Could you check a few things on this model? Use its own coordinates, in mm. Face numbers are marked on the shaded views. A direction names the side the tool comes from. Give positions to 0.01 mm unless a question says otherwise; leave off trailing zeros. Order: outer loops, then holes, each group sorted by start corner. A loop starts at its lowest first (then second) coordinate and runs counter-clockwise, first axis right, second up. Notation, with made-up numbers: M 61,-27 L 79,-27 A18 cw 79,1 Z; hole C 45,0 d10. An arc over 180 degrees is marked long. Use a Markdown table: item, result. Add a question column.
Item 1: Suppose I cut it at D-D on x = 10.5. Write out the boundary of the cut face in (y, z).
Item 2: I'm going to push flat-ended pins straight in: pin 1 Ø0.5 at (x, y) = (0, -3) entering from +Z; pin 2 Ø8 at (x, y) = (-1.5, -1.5) entering from -Z; pin 3 Ø2.5 at (x, y) = (0.5, 8.5) entering from +Z; pin 4 Ø1.2 at (x, y) = (0, -2.5) entering from +Z. Where does each tip first touch, or does it pass through?
Item 3: If I drill on L1, parallel to Y at x = 10.5, z = 0.7; L2, parallel to Z at x = 0.75, y = 6.25; L3, parallel to Y at x = -5.75, z = -0.2, over which ranges is the centre line in solid material (lowest first)? Write a range as from..to.
Item 4: Suppose I cut it at C-C on y = -4.5. Write out the boundary of the cut face in (x, z).
Item 5: Suppose I cut it at A-A on y = 3.25. Write out the boundary of the cut face in (x, z).
Item 6: For the marked faces 1, 2 and 3, which set-ups out of +Z, -Z, +X, -X, +Y, -Y let a thin tool reach every point of the face, with its end or its side?
Item 7: If we mould it in two halves opening along Y, with no side actions, what happens to the marked faces 4, 5 and 6? For each: released by +Y, released by -Y, zero draft, split by the parting line, or undercut.
Item 8: Suppose I cut it at B-B on x = 1.5. Write out the boundary of the cut face in (y, z) (3 decimals), plus the area to 3 significant figures.
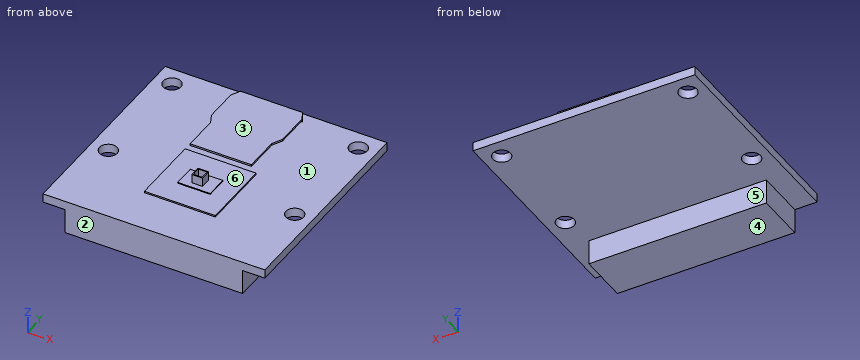
from build123d import *

# Parameters (mm, degrees)
SKETCH1_W                 = 25
SKETCH1_H                 = 24
BOSS_EXTRUDE1_DEPTH       = 1
SKETCH2_R                 = 1
CUT_EXTRUDE1_DEPTH        = 1
SKETCH3_W                 = 8
SKETCH3_H                 = 8
BOSS_EXTRUDE2_DEPTH       = 5.2
SKETCH4_W                 = 8
SKETCH4_H                 = 8
SKETCH4_R                 = 3.75
CUT_EXTRUDE2_DEPTH        = 3.2
SKETCH5_R                 = 3.75
SKETCH5_R_2               = 3
CUT_EXTRUDE3_DEPTH        = 1.2
TOP_RIBBON_DEPTH          = 1
SKETCH7_W                 = 0.8
SKETCH7_H                 = 9.7
CUT_EXTRUDE4_DEPTH        = 9
SKETCH8_W                 = 20
SKETCH8_H                 = 5.6
REAR_RIBBON_DEPTH         = 2.8
CUT_EXTRUDE5_DEPTH        = 10
CUT_EXTRUDE5_DEPTH_BACK   = 1.827942302
SKETCH9_W                 = 8
SKETCH9_H                 = 8
SKETCH10_W                = 3.67
SKETCH10_H                = 2.47
CCD_DEPTH                 = 0.1
SKETCH11_W                = 1.2
SKETCH11_H                = 1.2
SKETCH11_W_2              = 1
SKETCH11_H_2              = 1
TELESCOPE_ALIGNMENT_DEPTH = 1.1


with BuildPart() as part:
    # Sketch1 → Boss-Extrude1 (new body)
    with BuildSketch(Plane.XY):
        Rectangle(SKETCH1_W, SKETCH1_H)
    extrude(amount=BOSS_EXTRUDE1_DEPTH)

    # Sketch2 → Cut-Extrude1 (cut)
    with BuildSketch(Plane.XY.offset(1)):
        with Locations((-10.5, 9.85)):
            Circle(SKETCH2_R)
        with Locations((10.5, 9.85)):
            Circle(SKETCH2_R)
        with Locations((10.5, -2.65)):
            Circle(SKETCH2_R)
        with Locations((-10.5, -2.65)):
            Circle(SKETCH2_R)
    extrude(amount=-CUT_EXTRUDE1_DEPTH, mode=Mode.SUBTRACT)

    # Sketch3 → Boss-Extrude2 (add)
    with BuildSketch(Plane.XY.offset(1)):
        with Locations((0, -2.9)):
            Rectangle(SKETCH3_W, SKETCH3_H)
    extrude(amount=BOSS_EXTRUDE2_DEPTH)

    # Sketch4 → Cut-Extrude2 (cut)
    with BuildSketch(Plane.XY.offset(6.2)):
        with Locations((0, -2.9)):
            Rectangle(SKETCH4_W, SKETCH4_H)
        with Locations((0, -2.9)):
            Circle(SKETCH4_R, mode=Mode.SUBTRACT)
    extrude(amount=-CUT_EXTRUDE2_DEPTH, mode=Mode.SUBTRACT)

    # Sketch5 → Cut-Extrude3 (cut)
    with BuildSketch(Plane.XY.offset(6.2)):
        with Locations((0, -2.9)):
            Circle(SKETCH5_R)
        with Locations((0, -2.9)):
            Circle(SKETCH5_R_2, mode=Mode.SUBTRACT)
    extrude(amount=-CUT_EXTRUDE3_DEPTH, mode=Mode.SUBTRACT)

    # Sketch6 → Top Ribbon (add)
    with BuildSketch(Plane.XY.offset(1)):
        Polygon((-3.430481742, 1.1), (-3.430481742, 5.1), (-3.954291266, 6.2), (-3.954291266, 10), (-3.430481742, 11), (3.569518258, 11), (4.045708734, 10), (4.045708734, 6.2), (3.469518258, 5.1), (3.469518258, 1.1), align=None)
    extrude(amount=TOP_RIBBON_DEPTH)

    # Sketch7 → Cut-Extrude4 (cut)
    with BuildSketch(Plane(origin=(4.045708734, 0, 0), x_dir=(0, 0, -1), z_dir=(1, 0, 0))):
        with Locations((-1.4, 5.95)):
            Rectangle(SKETCH7_W, SKETCH7_H)
    extrude(amount=-CUT_EXTRUDE4_DEPTH, mode=Mode.SUBTRACT)

    # Sketch8 → Rear Ribbon (add)
    with BuildSketch(Plane(origin=(0, 0, 0), x_dir=(-1, 0, 0), z_dir=(0, 0, -1))):
        with Locations((0, -9.2)):
            Rectangle(SKETCH8_W, SKETCH8_H)
    extrude(amount=REAR_RIBBON_DEPTH)

    # Sketch9 → Cut-Extrude5 (cut, two sides: drawn at the far end of the back side and taken through both)
    with BuildSketch(Plane.XY.offset(3).offset(-CUT_EXTRUDE5_DEPTH_BACK)):
        with Locations((0, -2.9)):
            Rectangle(SKETCH9_W, SKETCH9_H)
    extrude(amount=CUT_EXTRUDE5_DEPTH + CUT_EXTRUDE5_DEPTH_BACK, mode=Mode.SUBTRACT)

    # Sketch10 → CCD (add)
    with BuildSketch(Plane.XY.offset(1.172057698)):
        with Locations((0, -2.9)):
            Rectangle(SKETCH10_W, SKETCH10_H)
    extrude(amount=CCD_DEPTH)

    # Sketch11 → Telescope Alignment (add)
    with BuildSketch(Plane.XY.offset(1.172057698)):
        with Locations((0, -2.9)):
            Rectangle(SKETCH11_W, SKETCH11_H)
        with Locations((0, -2.9)):
            Rectangle(SKETCH11_W_2, SKETCH11_H_2, mode=Mode.SUBTRACT)
    extrude(amount=TELESCOPE_ALIGNMENT_DEPTH)


solid = part.part
Findings below:
| question | item | result |
|---|---|---|
| 1 | outline | M -12,0 L -3.65,0 L -3.65,1 L -12,1 Z; M -1.65,0 L 8.85,0 L 8.85,1 L -1.65,1 Z; M 10.85,0 L 12,0 L 12,1 L 10.85,1 Z |
| 2 | pin 1 | stops at z = 1.27 |
| 2 | pin 2 | stops at z = 0 |
| 2 | pin 3 | stops at z = 2 |
| 2 | pin 4 | stops at z = 2.27 |
| 3 | L1 | y = -12..-3.65, -1.65..8.85, 10.85..12 |
| 3 | L2 | z = 0..1, 1.8..2 |
| 3 | L3 | y = -12..-6.4 |
| 4 | outline | M -12.5,0 L 12.5,0 L 12.5,1 L 4,1 L 4,1.17 L -4,1.17 L -4,1 L -12.5,1 Z |
| 5 | outline | M -12.5,0 L 12.5,0 L 12.5,1 L -12.5,1 Z; M -3.43,1.8 L 3.47,1.8 L 3.47,2 L -3.43,2 Z |
| 6 | face 1 | none |
| 6 | face 2 | +Z, -Z, +X, -X, -Y |
| 6 | face 3 | +Z, +X, -X, +Y |
| 7 | face 4 | zero draft |
| 7 | face 5 | released by +Y |
| 7 | face 6 | undercut |
| 8 | outline | M -12,-2.8 L -6.4,-2.8 L -6.4,0 L 12,0 L 12,1 L 11,1 L 11,2 L 1.1,2 L 1.1,1.8 L 10.8,1.8 L 10.8,1 L 1.1,1 L 1.1,1.172 L -1.665,1.172 L -1.665,1.272 L -4.135,1.272 L -4.135,1.172 L -6.9,1.172 L -6.9,1 L -12,1 Z |
| 8 | area | 43.4 mm^2 |
